from build123d import *

# Parameters (mm, degrees)
CROQUIS1_R              = 12
CROQUIS1_R_2            = 7.5
SALIENTE_EXTRUIR1_DEPTH = 2.5
CHAFL_N1_SIZE           = 0.5
CROQUIS2_R              = 10.711337482
CROQUIS2_R_2            = 9.016362729
SALIENTE_EXTRUIR2_DEPTH = 2.55


with BuildPart() as part:
    # Croquis1 → Saliente-Extruir1 (new body, symmetric)
    with BuildSketch(Plane(origin=(0, 0, 0), x_dir=(1, 0, 0), z_dir=(0, 1, 0))):
        Circle(CROQUIS1_R)
        Circle(CROQUIS1_R_2, mode=Mode.SUBTRACT)
    extrude(amount=SALIENTE_EXTRUIR1_DEPTH, both=True)

    # Chaflán1
    chafl_n1_edges = [part.edges().sort_by_distance(p)[0] for p in [
        (-12, -2.5, 0),
        (-12, 2.5, 0),
    ]]
    chamfer(chafl_n1_edges, length=CHAFL_N1_SIZE)

    # Croquis2 → Saliente-Extruir2 (add, symmetric)
    with BuildSketch(Plane(origin=(0, 0, 0), x_dir=(1, 0, 0), z_dir=(0, 1, 0))):
        Circle(CROQUIS2_R)
        Circle(CROQUIS2_R_2, mode=Mode.SUBTRACT)
    extrude(amount=SALIENTE_EXTRUIR2_DEPTH, both=True)


solid = part.part
Model file for the job. Use its own axes, mm. A direction names the side the tool comes from. Coordinates: 2 decimals unless noted, no trailing zeros. Order: outer loops, then holes, each group sorted by start corner. A loop starts at its lowest first (then second) coordinate and runs counter-clockwise, first axis right, second up. Notation, with made-up numbers: (86.25, 35.25) -> (95.25, 35.25) arc R8 ccw to (95.25, 44.25) -> close; hole circle Ø10 at (16, -29.5). An arc over 180 degrees is marked (long way). Return JSON: item names as keys, results as strings. Group by question number.
Item 1: Saw through at B-B on x = 0. Write the cut outline in (y, z).
Item 2: Flat gauge pins, fed straight in: P1, Ø9, axis at x = 0, z = 0, coming from the +Y side; P2, Ø1, axis at x = -4.5, y = -1.5, coming from the +Z side; P3, Ø1.5, axis at y = -1, z = 6.5, coming from the -X side. Where does each tip first touch, or does it go through?
Item 3: Wall check: line 1 along X through (y, z) = (0.95, -3.75); line 2 along X through (y, z) = (-2.45, 0); line 3 along Z through (x, y) = (1, -0.8). Give the ranges that are in metal, low to high. Write a range as [from, to].
Item 4: Saw through at A-A on z = 0. Write the cut outline in (x, y), then the cut area to 3 significant figures.
Item 5: Pull direction X, two halves, no side cores. Call faces 1 (the cylindrical face through (-7.493, -0.035, -0.33)), 2 (the cylindrical face through (-11.99, 0.03, -0.53)), 3 (the flat face through (-7.4, 2.5, 2)), 4 (the flat face through (-6, 2.55, 7)): pulls with the +X half, pulls with the -X half, needs draft (parallel to the pull), parting line crosses it, or undercut.
Item 6: Saw through at C-C on y = 0.05. Write the cut outline in (x, z), then the cut area to 3 significant figures.
Item 7: Tool access for faces 5 (the flat face through (-7.4, -2.5, 2)), 6 (the flat face through (-6, -2.55, 7)), 7 (the flat face through (8, 2.5, 8)): list every direction of +Z, -Z, +X, -X, +Y, -Y with a clear straight run to the whole face (end or side of a thin tool).
Values found:
{
 "1": {"outline": "(-2.55, -10.71) -> (-2.5, -10.71) -> (-2.5, -11.5) -> (-2, -12) -> (2, -12) -> (2.5, -11.5) -> (2.5, -10.71) -> (2.55, -10.71) -> (2.55, -9.02) -> (2.5, -9.02) -> (2.5, -7.5) -> (-2.5, -7.5) -> (-2.5, -9.02) -> (-2.55, -9.02) -> close; (-2.55, 9.02) -> (-2.5, 9.02) -> (-2.5, 7.5) -> (2.5, 7.5) -> (2.5, 9.02) -> (2.55, 9.02) -> (2.55, 10.71) -> (2.5, 10.71) -> (2.5, 11.5) -> (2, 12) -> (-2, 12) -> (-2.5, 11.5) -> (-2.5, 10.71) -> (-2.55, 10.71) -> close"},
 "2": {"P1": "passes through", "P2": "stops at z = 11.31", "P3": "stops at x = -10.53"},
 "3": {"line 1": "x = [-11.4, -6.5], [6.5, 11.4]", "line 2": "x = [-11.55, -7.5], [7.5, 11.55]", "line 3": "z = [-11.96, -7.43], [7.43, 11.96]"},
 "4": {"outline": "(-12, -2) -> (-11.5, -2.5) -> (-10.71, -2.5) -> (-10.71, -2.55) -> (-9.02, -2.55) -> (-9.02, -2.5) -> (-7.5, -2.5) -> (-7.5, 2.5) -> (-9.02, 2.5) -> (-9.02, 2.55) -> (-10.71, 2.55) -> (-10.71, 2.5) -> (-11.5, 2.5) -> (-12, 2) -> close; (7.5, -2.5) -> (9.02, -2.5) -> (9.02, -2.55) -> (10.71, -2.55) -> (10.71, -2.5) -> (11.5, -2.5) -> (12, -2) -> (12, 2) -> (11.5, 2.5) -> (10.71, 2.5) -> (10.71, 2.55) -> (9.02, 2.55) -> (9.02, 2.5) -> (7.5, 2.5) -> close", "area": "44.8 mm2"},
 "5": {"face 1": "undercut", "face 2": "parting line crosses it", "face 3": "undercut", "face 4": "needs draft"},
 "6": {"outline": "circle Ø24 at (0, 0); hole circle Ø15 at (0, 0)", "area": "276 mm2"},
 "7": {"face 5": "-Y", "face 6": "+Z, -Z, +X, -X, -Y", "face 7": "+Y"}
}
